Answer from the drawing. Dimensions are ordinates in mm from the lowest x, y and z of the part. Give positions to 0.01 mm unless a question says otherwise; leave off trailing zeros. Loops run counter-clockwise (first coordinate to the right, second up) from the corner with the lowest first, then second, coordinate; pieces in that order, holes last. Notation, with made-up numbers: (56, 4.25) - (95, 4.25) arc R28 ccw to (95, 41.25) - close; hole circle Ø9 at (-8, 70.5). An arc over 180 degrees is marked (long way). Put each result on its own line as item: value. Start each with the question number.
1. Consider L1, parallel to Z at x = 50.8, y = 2.25; L2, parallel to Z at x = 55.5, y = 2.9; L3, parallel to X at y = 1.05, z = 19.5 (1 decimal). Determine where each line is inside the solid, lowest interval first. Write a range as from..to.
2. A cutting plane is placed at C-C, the plane y = 2. Determine the outline of the cut face in (x, z), plus the area to 3 significant figures.
3. Given pin 1 Ø10 at (x, z) = (50.8, 19.05) entering from +Y, flat-ended and moving along its own axis, determine where the tip first touches the part or whether it passes through.
4. A cutting plane is placed at D-D, the plane z = 28.5. Determine the outline of the cut face in (x, y) (1 decimal).
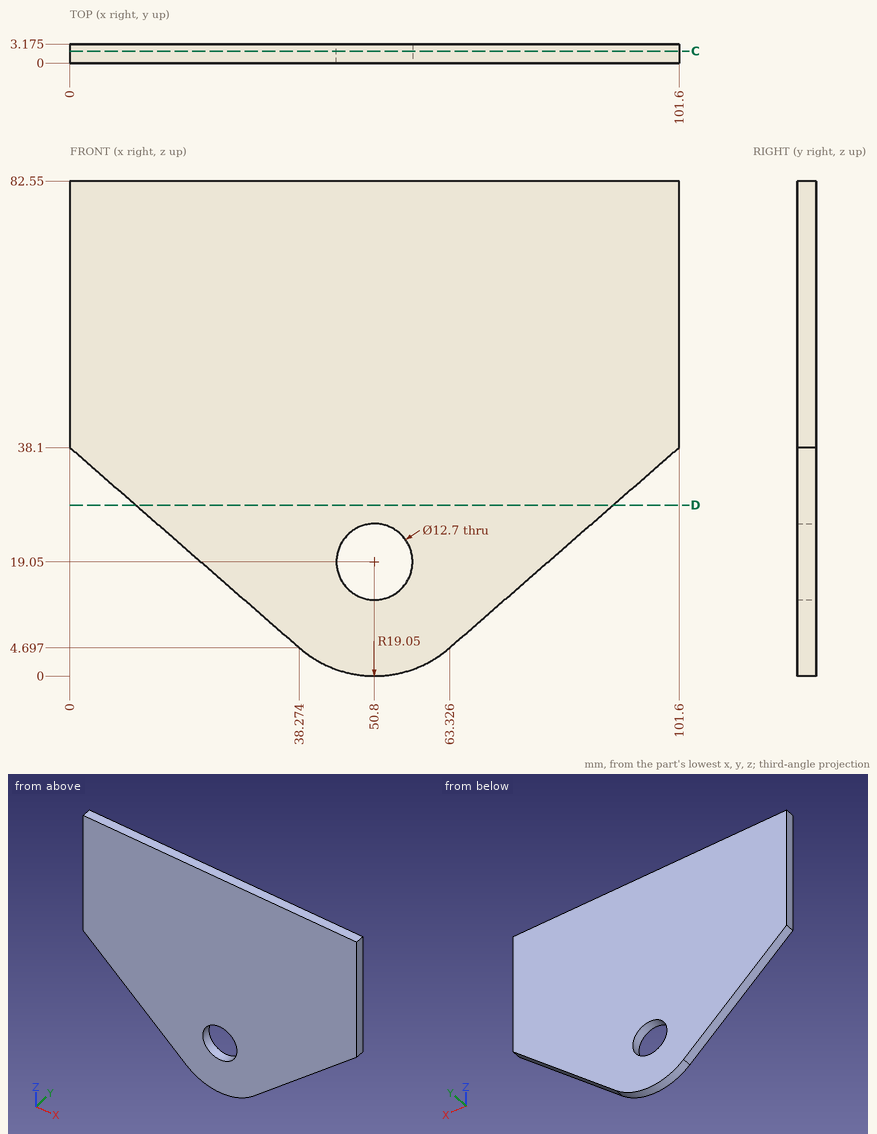
Return value:
1. L1: z = 0..12.7, 25.4..82.55
1. L2: z = 0.59..14.78, 23.32..82.55
1. L3: x = 21.3..44.5, 57.1..80.3
2. outline: (0, 38.1) - (38.27, 4.7) arc R19.05 ccw to (63.33, 4.7) - (101.6, 38.1) - (101.6, 82.55) - (0, 82.55) - close; hole circle Ø12.7 at (50.8, 19.05)
2. area: 6,590 mm2
3. pin 1: passes through
4. outline: (11, 0) - (90.6, 0) - (90.6, 3.2) - (11, 3.2) - close
